from build123d import *

# Parameters (mm, degrees)
SKETCH2_W           = 100
SKETCH2_H           = 150
BOSS_EXTRUDE1_DEPTH = 150
CUT_EXTRUDE1_DEPTH  = 235.520787991
CUT_EXTRUDE2_DEPTH  = 45


with BuildPart() as part:
    # Sketch2 → Boss-Extrude1 (new body)
    with BuildSketch(Plane(origin=(0, 0, 0), x_dir=(1, 0, 0), z_dir=(0, 1, 0))):
        with Locations((50, 75)):
            Rectangle(SKETCH2_W, SKETCH2_H)
    extrude(amount=BOSS_EXTRUDE1_DEPTH)

    # Sketch3 → Cut-Extrude1 (cut, through all)
    with BuildSketch(Plane.ZY):
        Polygon((0, 140), (-25, 140), (-140, 25), (-140, 0), (0, 0), align=None)
    extrude(amount=-CUT_EXTRUDE1_DEPTH, mode=Mode.SUBTRACT)

    # Sketch4 → Cut-Extrude2 (cut)
    with BuildSketch(Plane.ZY):
        Polygon((-140, 25), (-25, 140), (-140, 140), align=None)
    cut_extrude2 = extrude(amount=-CUT_EXTRUDE2_DEPTH, mode=Mode.SUBTRACT)

    # Mirror1: Cut-Extrude2 across plane
    add(cut_extrude2.mirror(Plane(origin=(50, 0, 0), x_dir=(0, 0, 1), z_dir=(1, 0, 0))), mode=Mode.SUBTRACT)


solid = part.part
Verification items for the finished model (mm, model axes). A direction names the side the tool comes from. Give positions to 0.01 mm unless a question says otherwise; leave off trailing zeros. Loops run counter-clockwise (first coordinate to the right, second up) from the corner with the lowest first, then second, coordinate; pieces in that order, holes last.
1. Go/stop test with flat-tipped pins: P1, Ø1.5, axis at x = 52, y = 30, coming from the +Z side; P2, Ø4, axis at x = 30, z = -19.5, coming from the -Y side; P3, Ø10, axis at y = 130.5, z = -99, coming from the +X side. Record where each tip stops, or that it passes through.
Derived:
P1: stops at z = -134.25
P2: stops at y = 140
P3: stops at x = 55
2. Cross-section at A-A on y = 112. Record the cut outline in (x, z), and give its area (3 significant figures).
Derived:
outline: (0, -150) - (100, -150) - (100, -140) - (55, -140) - (55, -53) - (45, -53) - (45, -140) - (0, -140) - close
area: 1,870 mm2
3. Material ranges on probe 1 along Z at (x, y) = (94.5, 80.5); probe 2 along Y at (x, z) = (44.5, -82.5); probe 3 along X at (y, z) = (122, -48), recorded low to high.
Derived:
probe 1: z = -150 to -140
probe 2: y = 140 to 150
probe 3: x = 45 to 55
4. Cross-section at B-B on x = 49.5. Record the cut outline in (y, z), and give its area (3 significant figures).
Derived:
outline: (0, -150) - (150, -150) - (150, 0) - (140, 0) - (140, -25) - (25, -140) - (0, -140) - close
area: 9,510 mm2
5. Cross-section at D-D on x = 27.5. Record the cut outline in (y, z), and give its area (3 significant figures).
Derived:
outline: (0, -150) - (150, -150) - (150, 0) - (140, 0) - (140, -140) - (0, -140) - close
area: 2,900 mm2
6. Cross-section at C-C on z = -52.5. Record the cut outline in (x, y), and give its area (4 significant figures).
Derived:
outline: (0, 140) - (45, 140) - (45, 112.5) - (55, 112.5) - (55, 140) - (100, 140) - (100, 150) - (0, 150) - close
area: 1,275 mm2
7. Tool access check on faces 1 (the flat face through (50, 83, -82)), 2 (the flat face through (55, 96, -96)), 3 (the flat face through (38, 140, -69)), 4 (the flat face through (49, 74, -150)), 5 (the flat face through (45, 96, -96)). Record the directions out of +Z, -Z, +X, -X, +Y, -Y that give a thin tool (end or side, any length) a straight path to the whole face; none if there is none.
Derived:
face 1: +Z, +X, -X, -Y
face 2: +Z, +X, -Y
face 3: +Z, -Y
face 4: -Z, +X, -X, +Y, -Y
face 5: +Z, -X, -Y
